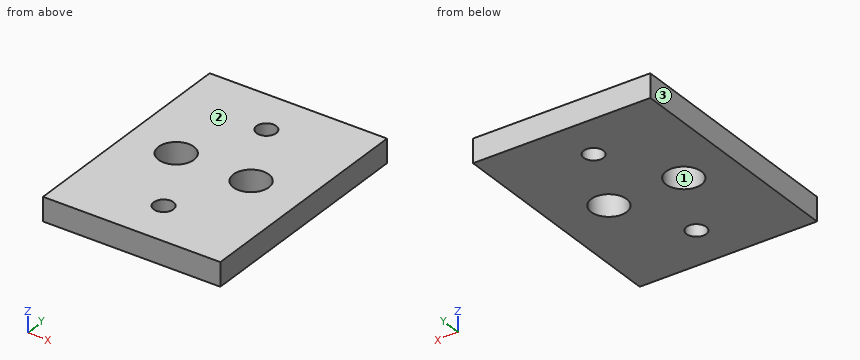
```python
from build123d import *

# Parameters (mm, degrees)
SKETCH1_W           = 45
SKETCH1_H           = 60
SKETCH1_R           = 4.5
SKETCH1_R_2         = 2.5
BOSS_EXTRUDE1_DEPTH = 6


with BuildPart() as part:
    # Sketch1 → Boss-Extrude1 (new body)
    with BuildSketch(Plane(origin=(0, 0, 0), x_dir=(-1, 0, 0), z_dir=(0, 0, -1))):
        Rectangle(SKETCH1_W, SKETCH1_H)
        with Locations(Location((-9.137137395, 0.033994069, 0), (0, 0, 180))):
            Circle(SKETCH1_R, mode=Mode.SUBTRACT)
        with Locations((0, 18.5)):
            Circle(SKETCH1_R_2, mode=Mode.SUBTRACT)
        with Locations((0, -18.5)):
            Circle(SKETCH1_R_2, mode=Mode.SUBTRACT)
        with Locations(Location((9.862862605, 0.033994069, 0), (0, 0, 180))):
            Circle(SKETCH1_R, mode=Mode.SUBTRACT)
    extrude(amount=-BOSS_EXTRUDE1_DEPTH)


solid = part.part
```
Read the model definition and answer for the solid it produces. Units are mm, in the model's axes. Face numbers are marked on the shaded views. Coordinates: 2 decimals unless noted, no trailing zeros. Write each loop counter-clockwise with the first axis right and the second up, starting at its lowest first coordinate (ties: lowest second). Pieces come first, ordered by that corner, then holes. Notation, with made-up numbers: (72, -31) - (125, -31) arc R22 ccw to (125, -18) - close; hole circle Ø4 at (30, 72.25). An arc over 180 degrees is marked (long way). Answer as a JSON object with one key per item and string values. Group by question number.
1. A cutting plane is placed at C-C (z = 4.95). Determine the outline of the cut face in (x, y), plus the area to 3 significant figures.
2. A cutting plane is placed at A-A (y = 18.5). Determine the outline of the cut face in (x, z), plus the area to 3 significant figures.
3. The mould has two halves that part along X. Classify the marked faces 1, 2 and 3: +X half, -X half, draft (parallel to the pull), parting line (faces both ways), or undercut.
4. A cutting plane is placed at D-D (y = -2.5). Determine the outline of the cut face in (x, z), plus the area to 3 significant figures.
5. Consider L1, parallel to Y at x = 0, z = 4.15; L2, parallel to Y at x = 1, z = 2.15; L3, parallel to X at y = -2, z = 3.8. Determine where each line is inside the solid, lowest interval first. Write a range as [from, to].
6. A cutting plane is placed at B-B (x = 0). Determine the outline of the cut face in (y, z), plus the area to 3 significant figures.
Worked out:
{
 "1": {"outline": "(-22.5, -30) - (22.5, -30) - (22.5, 30) - (-22.5, 30) - close; hole circle Ø9 at (-9.86, 0.03); hole circle Ø5 at (0, -18.5); hole circle Ø5 at (0, 18.5); hole circle Ø9 at (9.14, 0.03)", "area": "2,530 mm²"},
 "2": {"outline": "(-22.5, 0) - (-2.5, 0) - (-2.5, 6) - (-22.5, 6) - close; (2.5, 0) - (22.5, 0) - (22.5, 6) - (2.5, 6) - close", "area": "240 mm²"},
 "3": {"face 1": "undercut", "face 2": "draft", "face 3": "-X half"},
 "4": {"outline": "(-22.5, 0) - (-13.58, 0) - (-13.58, 6) - (-22.5, 6) - close; (-6.14, 0) - (5.42, 0) - (5.42, 6) - (-6.14, 6) - close; (12.86, 0) - (22.5, 0) - (22.5, 6) - (12.86, 6) - close", "area": "181 mm²"},
 "5": {"L1": "y = [-30, -21], [-16, 16], [21, 30]", "L2": "y = [-30, -20.79], [-16.21, 16.21], [20.79, 30]", "L3": "x = [-22.5, -13.88], [-5.85, 5.12], [13.15, 22.5]"},
 "6": {"outline": "(-30, 0) - (-21, 0) - (-21, 6) - (-30, 6) - close; (-16, 0) - (16, 0) - (16, 6) - (-16, 6) - close; (21, 0) - (30, 0) - (30, 6) - (21, 6) - close", "area": "300 mm²"}
}
